Work out the finished part from the listing and answer in its coordinate system (mm). Coordinates: 2 decimals unless noted, no trailing zeros. Order: outer loops, then holes, each group sorted by start corner. A loop starts at its lowest first (then second) coordinate and runs counter-clockwise, first axis right, second up.
```python
from build123d import *

# Parameters (mm, degrees)
SKETCH2_R                   = 9.525
BOSS_EXTRUDE1_DEPTH         = 1
M5_CLEARANCE_HOLE1_D        = 5.5
BOSS_EXTRUDE2_START         = -1.269999898
BOSS_EXTRUDE2_OUTLINE_R     = 9.525
BOSS_EXTRUDE2_OUTLINE_R_2   = 2.75
BOSS_EXTRUDE2_DEPTH         = 0.269999898
BOSS_EXTRUDE2_START_2       = 1.269999898
BOSS_EXTRUDE2_2_OUTLINE_R   = 9.525
BOSS_EXTRUDE2_2_OUTLINE_R_2 = 2.75
BOSS_EXTRUDE2_2_DEPTH       = 5.2217713
BOSS_EXTRUDE2_START_3       = -11
BOSS_EXTRUDE2_3_DEPTH       = 22
CUT_EXTRUDE1_DEPTH          = 15.546848663
CUT_EXTRUDE1_DEPTH_BACK     = 15.546848663


with BuildPart() as part:
    # Sketch2 → Boss-Extrude1 (new body)
    with BuildSketch(Plane(origin=(0, 0, 0), x_dir=(1, 0, 0), z_dir=(0, 1, 0))):
        with Locations(Location((0, 0, 0), (0, 0, 270))):
            Circle(SKETCH2_R)
    extrude(amount=BOSS_EXTRUDE1_DEPTH)

    # M5 Clearance Hole1 (through all)
    with Locations(Plane(origin=(0, 1, 0), x_dir=(1, 0, 0), z_dir=(0, 1, 0))):
        with Locations((0, 0)):
            Hole(M5_CLEARANCE_HOLE1_D / 2)

    # Boss-Extrude2: read off the stored shape, not the designer's step
    # Boss-Extrude2 outline → Boss-Extrude2 (add)
    with BuildSketch(Plane.XZ.offset(BOSS_EXTRUDE2_START)):
        Circle(BOSS_EXTRUDE2_OUTLINE_R)
        Circle(BOSS_EXTRUDE2_OUTLINE_R_2, mode=Mode.SUBTRACT)
    extrude(amount=BOSS_EXTRUDE2_DEPTH)

    # Boss-Extrude2 2 outline → Boss-Extrude2 2 (add)
    with BuildSketch(Plane(origin=(0, 0, 0), x_dir=(1, 0, 0), z_dir=(0, 1, 0)).offset(BOSS_EXTRUDE2_START_2)):
        Circle(BOSS_EXTRUDE2_2_OUTLINE_R)
        Circle(BOSS_EXTRUDE2_2_OUTLINE_R_2, mode=Mode.SUBTRACT)
    extrude(amount=BOSS_EXTRUDE2_2_DEPTH)

    # Boss-Extrude2 3 outline → Boss-Extrude2 3 (cut)
    with BuildSketch(Plane(origin=(0, 0, 0), x_dir=(0.51884630524159, 0, -0.8548675403459595), z_dir=(0.8548675403459595, 0, 0.5188463052415904)).offset(BOSS_EXTRUDE2_START_3)):
        with BuildLine():
            ThreePointArc((-9.525000037, 6.491771171), (-0.383965362, 1.319816038), (9.525621352, 4.799431821))
            Line((9.525621352, 4.799431821), (11, 6.211953819))
            Line((11, 6.211953819), (11, 6.491771198))
            Line((11, 6.491771198), (-9.525000037, 6.491771171))
        make_face()
    extrude(amount=BOSS_EXTRUDE2_3_DEPTH, mode=Mode.SUBTRACT)

    # Sketch7 → Cut-Extrude1 (cut, two sides: drawn at the far end of the back side and taken through both)
    with BuildSketch(Plane(origin=(0, 1, 0), x_dir=(1, 0, 0), z_dir=(0, 1, 0)).offset(-CUT_EXTRUDE1_DEPTH_BACK)):
        Polygon((-5.757007623, 7.588312608), (-9.388931759, 1.604239825), (-9.95857539, 1.949974666), (-6.326651253, 7.934047449), align=None)
    extrude(amount=CUT_EXTRUDE1_DEPTH + CUT_EXTRUDE1_DEPTH_BACK, mode=Mode.SUBTRACT)


solid = part.part
```
1. The part is cut by section B-B (y = 4.75). Determine the outline of the cut face in (x, z) (3 decimals).
2. Consider probe 1 along Z at (x, y) = (0, 0.85) (3 decimals); probe 2 along X at (y, z) = (1, -1.25). Determine where each line is inside the solid, lowest interval first.
3. The part is cut by section A-A (y = 3.5). Determine the outline of the cut face in (x, z) (3 decimals).
4. The mould has two halves that part along X. Classify faces 1 (the cylindrical face through (-0.181, 0.672, 2.744)), 2 (the flat face through (-7.548, 0.763, -4.638)), 3 (the flat face through (2.3, 0, 2)): released by +X, released by -X, zero draft, split by the parting line, or undercut.
5. The part is cut by section C-C (y = 6). Determine the outline of the cut face in (x, z) (3 decimals), plus the area to 3 significant figures.
6. Flat-ended cylindrical pins translate along their axes: pin 1 (1.5 mm diameter, centred on y = 2, z = -4, fed in from +X); pin 2 (1 mm diameter, centred on x = -6, z = -0.5, fed in from +Y); pin 3 (1 mm diameter, centred on x = -1, y = 3.5, fed in from +Z). Find the tip coordinate at first contact, or state that the pin passes through.
Worked out:
1. outline: (-8.575, 4.147) - (0.279, 9.521) arc R9.525 ccw to start; (4.072, -8.611) arc R9.525 ccw to (5.759, -7.587) - close
2. probe 1: z = -9.525 to -2.75, 2.75 to 9.525
2. probe 2: x = -9.44 to -2.45, 2.45 to 9.44
3. outline: (-9.339, 1.875) - (2.647, 9.15) arc R9.525 ccw to start; (-0.4, -9.517) arc R9.525 ccw to (8.627, -4.038) - close
4. face 1: undercut
4. face 2: released by -X
4. face 3: zero draft
5. outline: (-7.015, 6.444) - (-2.478, 9.197) arc R9.525 ccw to start
5. area: 1.34 mm2
6. pin 1: stops at x = 8.95
6. pin 2: stops at y = 1.89
6. pin 3: stops at z = 9.51
